```python
from build123d import *

# Parameters (mm, degrees)
PIPE_TAP_DRILL_FOR_3_8_TAP1_D     = 14.2748
PIPE_TAP_DRILL_FOR_3_8_TAP1_DEPTH = 25.4
PIPE_TAP_DRILL_FOR_3_8_TAP1_TIP   = 4.288582582
CIRPATTERN1_COUNT                 = 4


with BuildPart() as part:
    # Sketch1 → Revolve1 (revolve)
    with BuildSketch(Plane.XY):
        Polygon((-31.75, 0), (-15.875, 0), (-15.875, -63.5), (0, -63.5), (0, -73.025), (-22.225, -73.025), (-22.225, -6.35), (-31.75, -6.35), align=None)
    revolve(axis=Axis((0, 0, 0), (0, -1, 0)))

    # Pipe Tap Drill for 3/8 Tap1
    with Locations(Plane(origin=(0, -73.025, 0), x_dir=(-1, 0, 0), z_dir=(0, -1, 0))):
        with Locations((0, 0)):
            Hole(PIPE_TAP_DRILL_FOR_3_8_TAP1_D / 2, depth=PIPE_TAP_DRILL_FOR_3_8_TAP1_DEPTH)
            with Locations((0, 0, -(PIPE_TAP_DRILL_FOR_3_8_TAP1_DEPTH + PIPE_TAP_DRILL_FOR_3_8_TAP1_TIP / 2))):  # 118° drill point
                Cone(0, PIPE_TAP_DRILL_FOR_3_8_TAP1_D / 2, PIPE_TAP_DRILL_FOR_3_8_TAP1_TIP, mode=Mode.SUBTRACT)

    # Sketch3 → #10 Clearance Hole1 (revolve, cut)
    with BuildSketch(Plane(origin=(19.083044257, 0, -19.083044257), x_dir=(0, 0, 1), z_dir=(1, 0, 0))):
        Polygon((0, 0), (0, 26.933816902), (2.5527, 25.4), (2.5527, 0), align=None)
    f_10_clearance_hole1 = revolve(axis=Axis((19.083044257, 6.35, -19.083044257), (0, -1, 0)), mode=Mode.SUBTRACT)

    # CirPattern1: #10 Clearance Hole1 ×4 about axis
    cirpattern1_axis = Axis((0, 0, 0), (0, 1, 0))
    for i in range(1, CIRPATTERN1_COUNT):
        add(f_10_clearance_hole1.rotate(cirpattern1_axis, i * 360 / CIRPATTERN1_COUNT), mode=Mode.SUBTRACT)


solid = part.part
```
Geometry: final body of the model. Coordinates: model frame, mm. A direction names the side the tool comes from. Round coordinates to 2 decimals unless told otherwise and drop trailing zeros. Order: outer loops, then holes, each group sorted by start corner. A loop starts at its lowest first (then second) coordinate and runs counter-clockwise, first axis right, second up. Notation, with made-up numbers: (38.25, -10) - (56.25, -10) arc R34 cw to (56.25, 22) - close; hole circle Ø4 at (12.5, 85.25). An arc over 180 degrees is marked (long way). Write item = value, one per line. Start each with the question number.
Q1. Cut plane C-C on x = 18. Return the cut outline in (y, z) (3 decimals), and give its area (3 significant figures).
Q2. Pull-direction query (X, two-part tool) for faces 4 (the cylindrical face through (-21.199, -39.221, -6.676)), 5 (the cylindrical face through (-20.061, -3.131, 16.725)), 6 (the flat face through (-5.3, -73.025, -5.3)), 7 (the cylindrical face through (3.441, -32.194, 15.497)); classes: +X half, -X half, draft (parallel to the pull), parting line (faces both ways), or undercut.
Q3. Cut plane D-D on y = -16. Return the cut outline in (x, z) (3 decimals).
Q4. Cut plane B-B on x = 0. Return the cut outline in (y, z) (3 decimals).
Q5. Cut plane A-A on z = 0. Return the cut outline in (x, y) (3 decimals).
Q6. Ray query, line 1 (Z direction, x = 0, y = -21) (3 decimals); line 2 (Y direction, x = -26, z = -14); line 3 (X direction, y = -23, z = -7.5). Return the intervals inside material, ascending. Write a range as from..to.
Q7. Access query for faces 1 (the flat face through (-7, 0, -15)), 2 (the flat face through (-7, -63.5, 3)), 3 (the flat face through (-8, -6.35, -22)). Directions: +Z, -Z, +X, -X, +Y, -Y. A direction counts if a zero-diameter tool reaches every point of the face in a straight line with its end or side. Return the directions, or none.
Q8. Pin query (flat end, axial travel): pin 1 (8 mm diameter, centred on x = -19.08, z = 19.08, fed in from -Y); pin 2 (10 mm diameter, centred on x = -12, y = -46.5, fed in from -Z); pin 3 (4 mm diameter, centred on x = -19.08, z = -19.08, fed in from +Y); pin 4 (23 mm diameter, centred on x = 0, z = 0, fed in from -Y) (3 decimals). Return the tip coordinate at first contact, or that it passes through.
Outcome:
q1.outline = (-73.025, -13.037) - (-6.35, -13.037) - (-6.35, -16.771) - (0, -16.771) - (0, 16.771) - (-6.35, 16.771) - (-6.35, 13.037) - (-73.025, 13.037) - close; (-6.35, -26.155) - (0, -26.155) - (0, -21.395) - (-6.35, -21.395) - close; (-6.35, 21.395) - (0, 21.395) - (0, 26.155) - (-6.35, 26.155) - close
q1.area = 2,010 mm^2
q2.face_4 = parting line
q2.face_5 = undercut
q2.face_6 = draft
q2.face_7 = undercut
q3.outline = circle Ø44.45 at (0, 0); hole circle Ø31.75 at (0, 0)
q4.outline = (-73.025, -22.225) - (-6.35, -22.225) - (-6.35, -31.75) - (0, -31.75) - (0, -15.875) - (-63.5, -15.875) - (-63.5, -7.137) - (-73.025, -7.137) - close; (-73.025, 7.137) - (-63.5, 7.137) - (-63.5, 15.875) - (0, 15.875) - (0, 31.75) - (-6.35, 31.75) - (-6.35, 22.225) - (-73.025, 22.225) - close
q5.outline = (-31.75, -6.35) - (-22.225, -6.35) - (-22.225, -73.025) - (-7.137, -73.025) - (-7.137, -63.5) - (-15.875, -63.5) - (-15.875, 0) - (-31.75, 0) - close; (7.137, -73.025) - (22.225, -73.025) - (22.225, -6.35) - (31.75, -6.35) - (31.75, 0) - (15.875, 0) - (15.875, -63.5) - (7.137, -63.5) - close
q6.line_1 = -22.225..-15.875, 15.875..22.225
q6.line_2 = -6.35..0
q6.line_3 = -20.92..-13.99, 13.99..20.92
q7.face_1 = +Z, -Z, +X, -X, +Y
q7.face_2 = +Y
q7.face_3 = -Y
q8.pin_1 = -6.35
q8.pin_2 = -21.09
q8.pin_3 = through
q8.pin_4 = -73.025
